Design review of the part built by this model. Coordinates are the model's own, in mm. Face numbers are marked on the shaded views. A direction names the side the tool comes from. Coordinates: 2 decimals unless noted, no trailing zeros. Loops run counter-clockwise (first coordinate to the right, second up) from the corner with the lowest first, then second, coordinate; pieces in that order, holes last. Notation, with made-up numbers: (18, 54.25) - (44, 54.25) arc R14 cw to (44, 77.25) - close; hole circle Ø10 at (58.5, 31.25). An arc over 180 degrees is marked (long way). Return JSON: item names as keys, results as strings. Group by question number.
from build123d import *

# Parameters (mm, degrees)
SM_BASE_FLANGE_1_DEPTH = 40
CUT_EXTRUDE_1_REACH    = 195.197
SKETCH_6_R             = 7
CUT_EXTRUDE_2_REACH    = 274.213
SKETCH_7_R             = 7


# Sheet-metal steps are written as plain solids
with BuildPart() as part:
    # Sketch 1 → 基体-法兰1 (new body)
    with BuildSketch(Plane(origin=(0, 0, 0), x_dir=(1, 0, 0), z_dir=(0, 1, 0))):
        with BuildLine():
            Line((-105, 140), (-105, 4))
            ThreePointArc((-105, 4), (-103.828427125, 1.171572875), (-101, 0))
            Line((-101, 0), (101, 0))
            ThreePointArc((101, 0), (103.828427125, 1.171572875), (105, 4))
            Line((105, 4), (105, 140))
            Line((105, 140), (115, 140))
            Line((115, 140), (115, 4))
            ThreePointArc((115, 4), (110.899494937, -5.899494937), (101, -10))
            Line((101, -10), (-101, -10))
            ThreePointArc((-101, -10), (-110.899494937, -5.899494937), (-115, 4))
            Line((-115, 4), (-115, 140))
            Line((-115, 140), (-105, 140))
        make_face()
    extrude(amount=SM_BASE_FLANGE_1_DEPTH)

    # 草图6 → 切除-拉伸1 (cut, up to next)
    with BuildSketch(Plane.XY.offset(10), mode=Mode.PRIVATE) as cut_extrude_1_sk1:
        with Locations((-65, 20)):
            Circle(SKETCH_6_R)
    cut_extrude_1_tool1 = extrude(cut_extrude_1_sk1.sketch, amount=-CUT_EXTRUDE_1_REACH, mode=Mode.PRIVATE) & part.part
    # 草图6 → 切除-拉伸1 (cut, up to next)
    with BuildSketch(Plane.XY.offset(10), mode=Mode.PRIVATE) as cut_extrude_1_sk2:
        with Locations((65, 20)):
            Circle(SKETCH_6_R)
    cut_extrude_1_tool2 = extrude(cut_extrude_1_sk2.sketch, amount=-CUT_EXTRUDE_1_REACH, mode=Mode.PRIVATE) & part.part
    add(cut_extrude_1_tool1.solids().sort_by_distance((-65, 20, 10))[0], mode=Mode.SUBTRACT)
    add(cut_extrude_1_tool2.solids().sort_by_distance((65, 20, 10))[0], mode=Mode.SUBTRACT)

    # 切除-拉伸2: up to this face of the body (flat: up to its plane)
    cut_extrude_2_end = Plane(part.part.faces().sort_by_distance((-115, 20, -72))[0])
    # 草图7 → 切除-拉伸2 (cut, up to the picked face)
    with BuildSketch(Plane(origin=(115, 0, 0), x_dir=(0, 0, -1), z_dir=(1, 0, 0)), mode=Mode.PRIVATE) as cut_extrude_2_sk1:
        with Locations((122, 20)):
            Circle(SKETCH_7_R)
    cut_extrude_2_tool1 = split(extrude(cut_extrude_2_sk1.sketch, amount=-CUT_EXTRUDE_2_REACH, mode=Mode.PRIVATE), bisect_by=cut_extrude_2_end, keep=Keep.BOTH, mode=Mode.PRIVATE)
    # 草图7 → 切除-拉伸2 (cut, up to the picked face)
    with BuildSketch(Plane(origin=(115, 0, 0), x_dir=(0, 0, -1), z_dir=(1, 0, 0)), mode=Mode.PRIVATE) as cut_extrude_2_sk2:
        with Locations((72, 20)):
            Circle(SKETCH_7_R)
    cut_extrude_2_tool2 = split(extrude(cut_extrude_2_sk2.sketch, amount=-CUT_EXTRUDE_2_REACH, mode=Mode.PRIVATE), bisect_by=cut_extrude_2_end, keep=Keep.BOTH, mode=Mode.PRIVATE)
    # 草图7 → 切除-拉伸2 (cut, up to the picked face)
    with BuildSketch(Plane(origin=(115, 0, 0), x_dir=(0, 0, -1), z_dir=(1, 0, 0)), mode=Mode.PRIVATE) as cut_extrude_2_sk3:
        with Locations((22, 20)):
            Circle(SKETCH_7_R)
    cut_extrude_2_tool3 = split(extrude(cut_extrude_2_sk3.sketch, amount=-CUT_EXTRUDE_2_REACH, mode=Mode.PRIVATE), bisect_by=cut_extrude_2_end, keep=Keep.BOTH, mode=Mode.PRIVATE)
    add(cut_extrude_2_tool1.solids().sort_by(Axis((115, 20, -122), (-1, 0, 0)))[0], mode=Mode.SUBTRACT)
    add(cut_extrude_2_tool2.solids().sort_by(Axis((115, 20, -72), (-1, 0, 0)))[0], mode=Mode.SUBTRACT)
    add(cut_extrude_2_tool3.solids().sort_by(Axis((115, 20, -22), (-1, 0, 0)))[0], mode=Mode.SUBTRACT)


solid = part.part
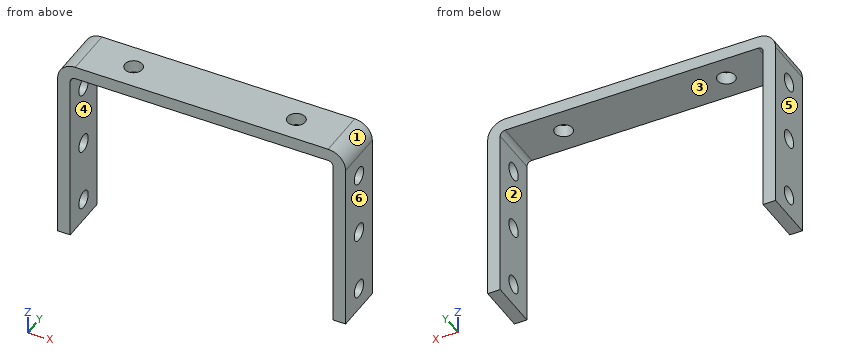
Item 1: To check wall thickness, follow line 1 (Y direction, x = 111, z = -22); line 2 (X direction, y = 9, z = -82); line 3 (Z direction, x = -6, y = 6). State the ranges of each line that lie inside material, in increasing order. Write a range as from..to.
Item 2: Add section A-A (z = -58). State the section outline as (x, y) points.
Item 3: For P1, Ø8.5, axis at y = 20, z = -22, coming from the -X side; P2, Ø2, axis at x = -46, y = 17, coming from the -Z side, all flat-tipped, find the tip position at first contact; note any pin that passes through.
Item 4: Add section B-B (x = 65). State the section outline as (y, z) points.
Item 5: For the marked faces 1 and 2, list the 3-axis set-ups (+Z, -Z, +X, -X, +Y, -Y) from which the entire face can be reached by the end or side of a thin tool; tool diameter is ignored.
Item 6: Add section C-C (z = -20.5). State the section outline as (x, y) points.
Item 7: Draft analysis for pull direction X (two halves, no side actions). For the marked faces 3, 4, 5 and 6, state which applies: pulls with the +X half, pulls with the -X half, needs draft (parallel to the pull), parting line crosses it, or undercut.
Item 8: Add section D-D (y = 30.5). State the section outline as (x, z) points.
Answers below:
{
 "1": {"line 1": "y = 0..13, 27..40", "line 2": "x = -115..-105, 105..115", "line 3": "z = 0..10"},
 "2": {"outline": "(-115, 0) - (-105, 0) - (-105, 40) - (-115, 40) - close; (105, 0) - (115, 0) - (115, 40) - (105, 40) - close"},
 "3": {"P1": "passes through", "P2": "stops at z = 0"},
 "4": {"outline": "(0, 0) - (13, 0) - (13, 10) - (0, 10) - close; (27, 0) - (40, 0) - (40, 10) - (27, 10) - close"},
 "5": {"face 1": "+Z, +X, +Y, -Y", "face 2": "-Z, +Y, -Y"},
 "6": {"outline": "(-115, 0) - (-105, 0) - (-105, 13.16) - (-115, 13.16) - close; (-115, 26.84) - (-105, 26.84) - (-105, 40) - (-115, 40) - close; (105, 0) - (115, 0) - (115, 13.16) - (105, 13.16) - close; (105, 26.84) - (115, 26.84) - (115, 40) - (105, 40) - close"},
 "7": {"face 3": "undercut", "face 4": "undercut", "face 5": "pulls with the -X half", "face 6": "pulls with the +X half"},
 "8": {"outline": "(-115, -140) - (-105, -140) - (-105, -4) arc R4 cw to (-101, 0) - (101, 0) arc R4 cw to (105, -4) - (105, -140) - (115, -140) - (115, -4) arc R14 ccw to (101, 10) - (-101, 10) arc R14 ccw to (-115, -4) - close"}
}
